Read the model definition and answer for the solid it produces. Units are mm, in the model's axes. A direction names the side the tool comes from. Coordinates: 2 decimals unless noted, no trailing zeros. Write each loop counter-clockwise with the first axis right and the second up, starting at its lowest first coordinate (ties: lowest second). Pieces come first, ordered by that corner, then holes. Notation, with made-up numbers: (-32, -22) -> (-9, -22) arc R21 ccw to (-9, 14) -> close; hole circle Ø7 at (-34.75, 86). An arc over 180 degrees is marked (long way). Return JSON: item names as keys, results as strings.
Autodesk Inventor part; units mm, degrees
ref_plane "YZ Plane" through (0, 0, 0) normal (1, 0, 0) x (0, 1, 0)
ref_plane "XZ Plane" through (0, 0, 0) normal (0, 1, 0) x (-1, 0, 0)
ref_plane "XY Plane" through (0, 0, 0) normal (0, 0, 1) x (1, 0, 0)
sketch "Sketch1" plane through (0, 0, 0) normal (1, 0, 0) x (0, 1, 0)
  line L0 (0, -112.9926) -> (0, 18.8321)
  line L1 (-133.1321, 0) -> (87.5926, 0)
  line L2 (0, 0) -> (50.8, 0)
  line L3 (50.8, 0) -> (50.8, -63.5)
  line L4 (25.4, -88.9) -> (-101.6, -88.9)
  line L5 (-101.6, -88.9) -> (-101.6, -63.5)
  line L6 (-101.6, -63.5) -> (-9.652, -63.5)
  line L7 (0, 0) -> (0, -53.848)
  arc A0 (25.4, -88.9) -> (50.8, -63.5) centre (25.4, -63.5) ccw
  arc A1 (-9.652, -63.5) -> (0, -53.848) centre (-9.652, -53.848) ccw
  point P0 (50.8, -88.9)
  point P1 (0, -63.5)
  dimension "d0" = 50.8
  dimension "d1" = 88.9
  dimension "d2" = 152.4
  dimension "d3" = 25.4
  dimension "d4" = 25.4
  dimension "d5" = 9.652
extrude "Extrusion1" add sketch "Sketch1" against normal blind 24.8285
sketch "Sketch6" plane through (0, -101.6, -88.9) normal (0, 0, -1) x (-1, 0, 0)
  circle A0 centre (12.4142, 12.7) radius 4.953
  line L0 (0, 0) -> (24.8285, 0)
  point P0 (0, 101.6)
  point P1 (12.4142, 0)
  dimension "d16" = 9.906
  dimension "d17" = 12.7
extrude "Extrusion4" cut sketch "Sketch6" against normal through all
sketch "Sketch7" plane through (0, -101.6, -88.9) normal (0, 0, -1) x (-1, 0, 0)
  circle A0 centre (12.4142, 12.7) radius 7.1374
  circle A1 centre (12.4142, 12.7) radius 4.953
  point P0 (0, 101.6)
  dimension "d20" = 14.2748
extrude "Extrusion5" cut sketch "Sketch7" against normal blind 9.525
sketch "Sketch8" plane through (0, 0, 0) normal (0, 0, 1) x (1, 0, 0)
  line L0 (0, 0) -> (-24.8285, 0)
  line L1 (-6.35, 50.8) -> (-6.35, 0)
  line L2 (-18.4785, 50.8) -> (-18.4785, 0)
  line L3 (0, 25.4) -> (0, 50.8)
  line L4 (-6.35, 50.8) -> (0, 50.8)
  line L5 (0, 0) -> (0, -9.652)
  line L6 (0, 50.8) -> (0, 0)
  line L7 (0, 0) -> (-6.35, 0)
  line L8 (-24.8285, 50.8) -> (-18.4785, 50.8)
  line L9 (-24.8285, 0) -> (-18.4785, 0)
  line L10 (-24.8285, 0) -> (-24.8285, 50.8)
  line L11 (-18.4785, 50.8) -> (-6.35, 50.8)
  line L12 (0, 50.8) -> (-24.8285, 50.8)
  line L13 (-18.4785, 0) -> (-6.35, 0)
  line L14 (0, 0) -> (-24.8285, 0)
  dimension "d23" = 6.35
  dimension "d24" = 6.35
extrude "Extrusion6" cut sketch "Sketch8" against normal blind 15.875 contours L0 L2 L11 L1
sketch "Sketch9" plane through (-24.8285, 0, 0) normal (0, 0, 1) x (1, 0, 0)
  line L0 (6.35, 50.8) -> (0, 50.8)
  line L1 (24.8285, 50.8) -> (18.4785, 50.8)
  line L2 (24.8285, 0) -> (18.4785, 0)
  line L3 (6.35, 0) -> (0, 0)
  point P0 (3.175, 47.625)
  point P1 (21.6535, 47.625)
  point P2 (21.6535, 3.175)
  point P3 (3.175, 3.175)
  point P4 (3.175, 50.8)
  point P5 (21.6535, 50.8)
  point P6 (21.6535, 0)
  dimension "d27" = 3.175
  dimension "d28" = 3.175
hole "Hole1" at (-21.6535, 47.625, 0) at (-3.175, 47.625, 0) at (-3.175, 3.175, 0) at (-21.6535, 3.175, 0) direction (0, 0, -1) diameter 3.302 depth 11.1252 tip angle 118
sketch "Sketch10" plane through (0, 0, 0) normal (1, 0, 0) x (0, 0, -1)
  line L0 (0, 50.8) -> (0, 0)
  point P0 (26.9748, 25.4)
  point P1 (0, 25.4)
  dimension "d36" = 26.9748
hole "Hole2" at (0, 25.4, -26.9748) direction (-1, 0, 0) diameter 12.7 end through all counterbore diameter 29.718 counterbore depth 19.7104
properties part number "Ch7(5) Part 13 Column"
1. Consider L1, parallel to Y at x = -3.75, z = -26.5; L2, parallel to Z at x = -6, y = 25.4; L3, parallel to Z at x = -18, y = -42.5. Determine where each line is inside the solid, lowest interval first.
Taken from the geometry:
{"L1": "y = 0 to 10.55, 40.25 to 50.8", "L2": "z = -88.9 to -41.83, -12.12 to 0", "L3": "z = -88.9 to -63.5"}
2. Flat-ended cylindrical pins translate along their axes: pin 1 Ø2 at (x, z) = (-22, -43.5) entering from -Y; pin 2 Ø3.5 at (x, y) = (-10, 41.5) entering from +Z (3 decimals); pin 3 Ø24 at (y, z) = (25, -29) entering from +X; pin 4 Ø8 at (x, y) = (-12.41, -88.9) entering from -Z. Find the tip coordinate at first contact, or state that the pin passes through.
Taken from the geometry:
{"pin 1": "stops at y = 0", "pin 2": "stops at z = -15.875", "pin 3": "stops at x = -19.71", "pin 4": "passes through"}
3. The part is cut by section B-B (x = -15.75). Determine the outline of the cut face in (y, z) (3 decimals).
Taken from the geometry:
{"outline": "(-101.6, -88.9) -> (-95.21, -88.9) -> (-95.21, -79.375) -> (-92.561, -79.375) -> (-92.561, -63.5) -> (-101.6, -63.5) -> close; (-85.239, -79.375) -> (-82.59, -79.375) -> (-82.59, -88.9) -> (25.4, -88.9) arc R25.4 ccw to (50.8, -63.5) -> (50.8, -15.875) -> (35.278, -15.875) arc R14.859 cw (long way) to (15.522, -15.875) -> (0, -15.875) -> (0, -53.848) arc R9.652 cw to (-9.652, -63.5) -> (-85.239, -63.5) -> close"}
4. The part is cut by section C-C (z = -31). Determine the outline of the cut face in (x, y).
Taken from the geometry:
{"outline": "(-24.83, 0) -> (0, 0) -> (0, 11.1) -> (-19.71, 11.1) -> (-19.71, 20.49) -> (-24.83, 20.49) -> close; (-24.83, 30.31) -> (-19.71, 30.31) -> (-19.71, 39.7) -> (0, 39.7) -> (0, 50.8) -> (-24.83, 50.8) -> close"}
5. A tool of negligible diameter and unlimited length cuts with its end or side. For faces 1 (the face through (-18.478, 26, -8)), 2 (the face through (-11.485, -81.823, -84.204)), 3 (the face through (-12.24, -2.902, -60.748)), 4 (the face through (-23.046, 46.737, -5.64)), 5 (the face through (-24.828, -10, -64)), from which of +Z, -Z, +X, -X, +Y, -Y can it reach the whole face along a straight path? Write none if from no direction.
Taken from the geometry:
{"face 1": "+Z, +Y, -Y", "face 2": "-Z", "face 3": "+Z, +X, -X, -Y", "face 4": "+Z", "face 5": "+Z, -Z, -X, +Y, -Y"}
6. For a pull along Y with two mould halves and no side action, classify faces 6 (the face through (-21.369, 47.662, -11.945)), 7 (the face through (-12, 50.8, -31)), 8 (the face through (-12, -56, -63.5)) as +Y half, -Y half, draft (parallel to the pull), parting line (faces both ways), or undercut.
Taken from the geometry:
{"face 6": "undercut", "face 7": "+Y half", "face 8": "draft"}
7. The part is cut by section D-D (z = -81). Determine the outline of the cut face in (x, y).
Taken from the geometry:
{"outline": "(-24.83, -101.6) -> (0, -101.6) -> (0, 43.81) -> (-24.83, 43.81) -> close; hole circle Ø14.27 at (-12.41, -88.9)"}
8. The part is cut by section A-A (y = -88.9). Determine the outline of the cut face in (x, z) (1 decimal), then the cut area to 3 significant figures.
Taken from the geometry:
{"outline": "(-24.8, -88.9) -> (-19.6, -88.9) -> (-19.6, -79.4) -> (-17.4, -79.4) -> (-17.4, -63.5) -> (-24.8, -63.5) -> close; (-7.5, -79.4) -> (-5.3, -79.4) -> (-5.3, -88.9) -> (0, -88.9) -> (0, -63.5) -> (-7.5, -63.5) -> close", "area": "337 mm2"}
